```python
from build123d import *

# Parameters (mm, degrees)
SKIZZE2_W                       = 40
SKIZZE2_H                       = 17.5
SCHNITT_LINEAR_AUSTRAGEN1_DEPTH = 56.957573214
SKIZZE6_W                       = 2
SKIZZE6_H                       = 16.5
SCHNITT_LINEAR_AUSTRAGEN3_DEPTH = 56.957573214
SKIZZE10_R                      = 4
SCHNITT_LINEAR_AUSTRAGEN4_DEPTH = 11.5
KERNLOCH_F_R_M4_GEWINDE1_D      = 3.3


with BuildPart() as part:
    # Skizze2 → Rotation1 (revolve)
    with BuildSketch(Plane.XY, mode=Mode.PRIVATE) as rotation1_sk:
        with Locations((20, 8.75)):
            Rectangle(SKIZZE2_W, SKIZZE2_H)
    revolve(rotation1_sk.sketch.rotate(Axis((0, 17.5, 0), (1, 0, 0)), 270), axis=Axis((0, 17.5, 0), (1, 0, 0)))

    # Skizze3 → Schnitt-Linear austragen1 (cut, through all)
    with BuildSketch(Plane.ZY):
        with BuildLine():
            Line((5.408326913, 18.5), (19.826246022, 18.5))
            Line((19.826246022, 18.5), (19.826246022, 16.5))
            Line((19.826246022, 16.5), (5.408326913, 16.5))
            ThreePointArc((5.408326913, 16.5), (0, 12), (-5.408326913, 16.5))
            Line((-5.408326913, 16.5), (-8.5, 16.5))
            Line((-8.5, 16.5), (-8.5, 17.5))
            Line((-8.5, 17.5), (-8.5, 18.5))
            Line((-8.5, 18.5), (-5.408326913, 18.5))
            ThreePointArc((-5.408326913, 18.5), (0, 23), (5.408326913, 18.5))
        make_face()
    extrude(amount=-SCHNITT_LINEAR_AUSTRAGEN1_DEPTH, mode=Mode.SUBTRACT)

    # Skizze6 → Schnitt-Linear austragen3 (cut, through all)
    with BuildSketch(Plane.XY):
        with Locations((20, 8.25)):
            Rectangle(SKIZZE6_W, SKIZZE6_H)
        with Locations((20, 26.75)):
            Rectangle(SKIZZE6_W, SKIZZE6_H)
    extrude(amount=SCHNITT_LINEAR_AUSTRAGEN3_DEPTH, mode=Mode.SUBTRACT)

    # Skizze10 → Schnitt-Linear austragen4 (cut)
    with BuildSketch(Plane(origin=(0, 35, 0), x_dir=(1, 0, 0), z_dir=(0, 1, 0))):
        with Locations(Location((26, -11, 0), (0, 0, 270))):
            Circle(SKIZZE10_R)
        with Locations(Location((35, -11, 0), (0, 0, 270))):
            Circle(SKIZZE10_R)
        with Locations(Location((5, -11, 0), (0, 0, 270))):
            Circle(SKIZZE10_R)
        with Locations(Location((14, -11, 0), (0, 0, 270))):
            Circle(SKIZZE10_R)
    extrude(amount=-SCHNITT_LINEAR_AUSTRAGEN4_DEPTH, mode=Mode.SUBTRACT)

    # Kernloch für M4 Gewinde1 (through all)
    with Locations(Plane(origin=(5, 23.5, 11), x_dir=(0, 0, 1), z_dir=(0, 1, 0))):
        with Locations((0, 0), (0, 9), (0, 21), (0, 30)):
            Hole(KERNLOCH_F_R_M4_GEWINDE1_D / 2)


solid = part.part
```
Geometry: final body of the model. Coordinates: model frame, mm. A direction names the side the tool comes from. Round coordinates to 2 decimals unless told otherwise and drop trailing zeros. Loops run counter-clockwise (first coordinate to the right, second up) from the corner with the lowest first, then second, coordinate; pieces in that order, holes last. Notation, with made-up numbers: (22.25, -16) -> (72.25, -16) arc R22 ccw to (72.25, 3) -> close; hole circle Ø4 at (73.5, 52). An arc over 180 degrees is marked (long way). Use one line per item in the form item = value.
Item 1: Cut plane A-A on y = 20. Output: boundary loops of the cut face in (x, z), then the cut area to 3 significant figures.
Evaluation:
outline = (0, -17.32) -> (40, -17.32) -> (40, -4.9) -> (0, -4.9) -> close; (0, 4.9) -> (19, 4.9) -> (19, 17.32) -> (0, 17.32) -> close; (21, 4.9) -> (40, 4.9) -> (40, 17.32) -> (21, 17.32) -> close; hole circle Ø3.3 at (5, 11); hole circle Ø3.3 at (14, 11); hole circle Ø3.3 at (26, 11); hole circle Ø3.3 at (35, 11)
area = 935 mm2
Item 2: Access query for faces 1 (the flat face through (30, 18.5, 11)), 2 (the flat face through (20, 29, 0)), 3 (the flat face through (12, 23.5, 11)). Directions: +Z, -Z, +X, -X, +Y, -Y. A direction counts if a zero-diameter tool reaches every point of the face in a straight line with its end or side. Return the directions, or none.
Evaluation:
face_1 = +Z, +X, -X
face_2 = +Z, +Y, -Y
face_3 = +Y
Item 3: Cut plane B-B on x = 35. Output: boundary loops of the cut face in (y, z), then the cut area to 3 significant figures.
Evaluation:
outline = (2.71, 9.35) arc R17.5 ccw (long way) to (33.54, 7) -> (23.5, 7) -> (23.5, 9.35) -> (18.5, 9.35) -> (18.5, 5.41) arc R5.5 cw to (18.5, -5.41) -> (18.5, -8.5) -> (16.5, -8.5) -> (16.5, -5.41) arc R5.5 cw to (16.5, 5.41) -> (16.5, 9.35) -> close; (5.41, 12.65) -> (16.5, 12.65) -> (16.5, 17.47) arc R17.5 ccw to start; (18.5, 12.65) -> (23.5, 12.65) -> (23.5, 15) -> (26.51, 15) arc R17.5 ccw to (18.5, 17.47) -> close
area = 721 mm2
Item 4: Cut plane D-D on z = 4. Output: boundary loops of the cut face in (x, y).
Evaluation:
outline = (0, 0.46) -> (19, 0.46) -> (19, 13.73) -> (0, 13.73) -> close; (0, 21.27) -> (19, 21.27) -> (19, 34.54) -> (0, 34.54) -> close; (21, 0.46) -> (40, 0.46) -> (40, 13.73) -> (21, 13.73) -> close; (21, 21.27) -> (40, 21.27) -> (40, 34.54) -> (21, 34.54) -> close
Item 5: Material intervals for probe 1 along X at (y, z) = (22, 11); probe 2 along X at (y, z) = (27.75, 11); probe 3 along X at (y, z) = (22, 4), sorted ascending.
Evaluation:
probe_1 = 0 to 3.35, 6.65 to 12.35, 15.65 to 19, 21 to 24.35, 27.65 to 33.35, 36.65 to 40
probe_2 = 0 to 1, 9 to 10, 18 to 19, 21 to 22, 30 to 31, 39 to 40
probe_3 = 0 to 19, 21 to 40
Item 6: Draft query along Z for faces 4 (the flat face through (9, 16.5, 12)), 5 (the flat face through (20, 6, 0)), 6 (the cylindrical face through (35, 27, 7)), 7 (the flat face through (3, 23.5, 11)). Return one class per face: released by +Z, released by -Z, zero draft, split by the parting line, or undercut.
Evaluation:
face_4 = zero draft
face_5 = released by +Z
face_6 = undercut
face_7 = undercut
Item 7: Cut plane C-C on z = -7. Output: boundary loops of the cut face in (x, y), then the cut area to 3 significant figures.
Evaluation:
outline = (0, 1.46) -> (40, 1.46) -> (40, 16.5) -> (0, 16.5) -> close; (0, 18.5) -> (40, 18.5) -> (40, 33.54) -> (0, 33.54) -> close
area = 1,200 mm2
Item 8: Contact query for flat-ended pins moving along their axis: pin 1 Ø4 at (x, y) = (24, 9.5) entering from -Z; pin 2 Ø3 at (x, z) = (14, 11) entering from +Y; pin 3 Ø4 at (x, z) = (35.5, 10.5) entering from +Y; pin 4 Ø2 at (x, y) = (19.5, 28) entering from +Z. Output: stop coordinate, or through.
Evaluation:
pin_1 = -16.44
pin_2 = through
pin_3 = 23.5
pin_4 = 14.61
